```python
from build123d import *

# Parameters (mm, degrees)
EXTRUDE_1_DEPTH     = 90
SKETCH_2_R          = 2.75
CUT_EXTRUDE_1_DEPTH = 124.693168769


with BuildPart() as part:
    # Эскиз1 → Бобышка-Вытянуть1 (new body)
    with BuildSketch(Plane.XY):
        Polygon((0, 0), (0, 60), (3, 60), (3, 3), (60, 3), (60, 0), align=None)
    extrude(amount=EXTRUDE_1_DEPTH)

    # Эскиз2 → Вырез-Вытянуть1 (cut, through all)
    with BuildSketch(Plane.XZ):
        with Locations((10, 75)):
            Circle(SKETCH_2_R)
        with Locations((46, 75)):
            Circle(SKETCH_2_R)
        with Locations((46, 15)):
            Circle(SKETCH_2_R)
        with Locations((10, 15)):
            Circle(SKETCH_2_R)
    extrude(amount=-CUT_EXTRUDE_1_DEPTH, mode=Mode.SUBTRACT)


solid = part.part
```
Read the model definition and answer for the solid it produces. Units are mm, in the model's axes. A direction names the side the tool comes from. Round coordinates to 2 decimals unless told otherwise and drop trailing zeros. Write each loop counter-clockwise with the first axis right and the second up, starting at its lowest first coordinate (ties: lowest second). Pieces come first, ordered by that corner, then holes. Notation, with made-up numbers: (20.25, 48.25) - (72.25, 48.25) arc R30 ccw to (72.25, 81.25) - close; hole circle Ø4 at (-30.5, 37). An arc over 180 degrees is marked (long way). One line per item, written item: value.
Q1. Find section B-B (z = 15). Determine the outline of the cut face in (x, y), and give its area (3 significant figures).
The answers:
outline: (0, 0) - (7.25, 0) - (7.25, 3) - (3, 3) - (3, 60) - (0, 60) - close; (12.75, 0) - (43.25, 0) - (43.25, 3) - (12.75, 3) - close; (48.75, 0) - (60, 0) - (60, 3) - (48.75, 3) - close
area: 318 mm2
Q2. For a pull along X with two mould halves and no side action, classify faces 3 (the flat face through (0, 30, 44)), 4 (the cylindrical face through (43.253, 1.479, 15.121)), 5 (the flat face through (31, 3, 44)) as pulls with the +X half, pulls with the -X half, needs draft (parallel to the pull), parting line crosses it, or undercut.
The answers:
face 3: pulls with the -X half
face 4: undercut
face 5: needs draft
Q3. Find section A-A (x = 46). Determine the outline of the cut face in (y, z), and give its area (3 significant figures).
The answers:
outline: (0, 0) - (3, 0) - (3, 12.25) - (0, 12.25) - close; (0, 17.75) - (3, 17.75) - (3, 72.25) - (0, 72.25) - close; (0, 77.75) - (3, 77.75) - (3, 90) - (0, 90) - close
area: 237 mm2
Q4. Straight lines are drawn through the part: line 1 (Z direction, x = 10, y = 1); line 2 (Y direction, x = 27.5, z = 82.5). For each, find the intervals that lie inside material, in ascending order. Write a range as from..to.
The answers:
line 1: z = 0..12.25, 17.75..72.25, 77.75..90
line 2: y = 0..3
Q5. Find section C-C (z = 68). Determine the outline of the cut face in (x, y), and give its area (3 significant figures).
The answers:
outline: (0, 0) - (60, 0) - (60, 3) - (3, 3) - (3, 60) - (0, 60) - close
area: 351 mm2
Q6. Find section D-D (y = 16). Determine the outline of the cut face in (x, z), and give its area (3 significant figures).
The answers:
outline: (0, 0) - (3, 0) - (3, 90) - (0, 90) - close
area: 270 mm2
Q7. Each of these flat-tipped pins is pushed along its axis until it touches: P1, Ø7, axis at x = 46, z = 15, coming from the +Y side; P2, Ø1, axis at y = 50.5, z = 12, coming from the +X side; P3, Ø12, axis at y = 19.5, z = 18, coming from the -X side. Where does it stop, or does it pass through?
The answers:
P1: stops at y = 3
P2: stops at x = 3
P3: stops at x = 0
Q8. Which of the six approach directions +Z, -Z, +X, -X, +Y, -Y give full straight-line access (tool end or side, diameter ignored) to faces 1 (the cylindrical face through (43.973, 1.479, 76.859)), 2 (the flat face through (3, 32, 44))?
The answers:
face 1: +Y, -Y
face 2: +Z, -Z, +X, +Y
